Verification items for the finished model (mm, model axes). A direction names the side the tool comes from. Round coordinates to 2 decimals unless told otherwise and drop trailing zeros. Loops run counter-clockwise (first coordinate to the right, second up) from the corner with the lowest first, then second, coordinate; pieces in that order, holes last. Notation, with made-up numbers: (-20.5, -10.5) -> (10.5, -10.5) arc R29 ccw to (10.5, 10.5) -> close; hole circle Ø3 at (-33.75, 19.25). An arc over 180 degrees is marked (long way). Use a Markdown table: item, result. Add a question column.
```python
from build123d import *

# Parameters (mm, degrees)
BOSS_EXTRUDE1_DEPTH = 2


with BuildPart() as part:
    # Sketch1 → Boss-Extrude1 (new body)
    with BuildSketch(Plane(origin=(0, 0, 0), x_dir=(1, 0, 0), z_dir=(0, 1, 0))):
        Polygon((0, 0), (21.11421446, 0), (18.47519345, 15.619407395), (3.517557511, 20.81914603), align=None)
        Polygon((5.884430734, 16.82024507), (3.549392266, 3), (17.564822194, 3), (15.812934214, 13.368789015), align=None, mode=Mode.SUBTRACT)
    extrude(amount=BOSS_EXTRUDE1_DEPTH)


solid = part.part
```
1) Sectioned sample at D-D on z = -18. Enter the section's corners in (x, y).
2) Access from +Z, -Z, +X, -X, +Y, -Y to the whole of each face (thin tool, end or side, straight path). Record for faces 5 (the face through (3, 2, -8)), 6 (the face through (10.92, 0.99, -15.07)).
3) Sectioned sample at C-C on z = -10.5. Enter the section's corners in (x, y).
4) Go/stop test with a flat-tipped pin: pin 1 (4 mm diameter, centred on x = 15.5, z = -10.5, fed in from -Y). Record where the tip stops, or that it passes through.
5) Sectioned sample at A-A on x = 4. Enter the section's corners in (y, z).
6) Sectioned sample at B-B on y = 0.5. Enter the section's corners in (x, z), then the cut area to 3 significant figures.
7) Thickness scan on line 1 (Z direction, x = 13, y = 0.9); line 2 (X direction, y = 0.9, z = -9); line 3 (Z direction, x = 10.75, y = 1.3). Record the ranges inside material, lowest first.
8) Release check for a two-part mould opening along X. For faces 1 (the face through (1.783, 0.986, -10.555)), 2 (the face through (11.101, 0.986, -18.183)), 3 (the face through (10, 1, -3)), 4 (the face through (3, 0, -8)) record: released by +X, released by -X, zero draft, split by the parting line, or undercut.
Geometry results:
| question | item | result |
|---|---|---|
| 1 | outline | (3.04, 0) -> (11.63, 0) -> (11.63, 2) -> (3.04, 2) -> close |
| 2 | face 5 | +Z, -Z, +X, -X, +Y |
| 2 | face 6 | +Y, -Y |
| 3 | outline | (1.77, 0) -> (4.82, 0) -> (4.82, 2) -> (1.77, 2) -> close; (16.3, 0) -> (19.34, 0) -> (19.34, 2) -> (16.3, 2) -> close |
| 4 | pin 1 | y = 0 |
| 5 | outline | (0, -20.65) -> (2, -20.65) -> (2, -5.67) -> (0, -5.67) -> close; (0, -3) -> (2, -3) -> (2, 0) -> (0, 0) -> close |
| 6 | outline | (0, 0) -> (3.52, -20.82) -> (18.48, -15.62) -> (21.11, 0) -> close; hole (3.55, -3) -> (5.88, -16.82) -> (15.81, -13.37) -> (17.56, -3) -> close |
| 6 | area | 184 mm^2 |
| 7 | line 1 | -17.52 to -14.35, -3 to 0 |
| 7 | line 2 | 1.52 to 4.56, 16.55 to 19.59 |
| 7 | line 3 | -18.3 to -15.13, -3 to 0 |
| 8 | face 1 | released by -X |
| 8 | face 2 | released by +X |
| 8 | face 3 | undercut |
| 8 | face 4 | zero draft |
